For this review, take the finished solid that the model builds, in its own axes (mm). A direction names the side the tool comes from. Coordinates: 2 decimals unless noted, no trailing zeros. Order: outer loops, then holes, each group sorted by start corner. A loop starts at its lowest first (then second) coordinate and runs counter-clockwise, first axis right, second up. Notation, with made-up numbers: (84.25, -4) - (120.25, -4) arc R19 ccw to (120.25, 19) - close; hole circle Ø4 at (12, -7). An arc over 180 degrees is marked (long way). One line per item, written item: value. Start each with the question number.
(1) Consider section D-D on y = -26. Write out the cut boundary in (x, z).
(2) To check wall thickness, follow line 1 along Z through (x, y) = (-56.5, 14.5); line 2 along X through (y, z) = (1, 28); line 3 along X through (y, z) = (2, 11). State the ranges of each line that lie inside material, in increasing order.
(3) Consider section A-A on y = 0. Write out the cut boundary in (x, z).
(4) Consider section C-C on z = 21.5. Write out the cut boundary in (x, y), then the cut area to 3 significant figures.
(5) Consider section B-B on x = -55. Write out the cut boundary in (y, z), then the cut area to 3 significant figures.
(6) Clearance check with flat-ended pins moving along their axes: pin 1 (6 mm diameter, centred on x = 5, y = -17, fed in from -Z); pin 2 (21 mm diameter, centred on x = -18.5, y = 5.5, fed in from +Z); pin 3 (12 mm diameter, centred on y = -4.5, z = 22, fed in from +X). State where each tip first meets the part, or that it passes through.
(7) Mouldability with a two-part tool opening along Y and no side actions: class faces 1 (the flat face through (60, 0, 53.848)), 2 (the cylindrical face through (63.58, 0.98, 28.48)), 3 (the cylindrical face through (63.58, 0.98, 0.63)) as released by +Y, released by -Y, zero draft, split by the parting line, or undercut.
(8) For faces 4 (the flat face through (0, 5, 1.27)), 5 (the flat face through (0, 39.716, 2)), 6 (the cylindrical face through (-63.075, 0.142, 28.479)), list the 3-axis set-ups (+Z, -Z, +X, -X, +Y, -Y) from which the entire face can be reached by the end or side of a thin tool; tool diameter is ignored.
```python
from build123d import *

# Parameters (mm, degrees)
F0_W     = 134.956628
F0_H     = 69.98465
F1_DEPTH = 3.81
F2_T     = -2.54
F3_R     = 3.221336
F3_R_2   = 3.263541
F4_DEPTH = 53.848


with BuildPart() as f1:
    # F0 (on Top) → F1 (new body)
    with BuildSketch(Plane.XY):
        with Locations((1.349568, 4.723483)):
            Rectangle(F0_W, F0_H)
    extrude(amount=F1_DEPTH)

    # F2
    f2_openings = [f1.faces().sort_by_distance(p)[0] for p in [
        (1.349568, 4.723483, 0),
    ]]
    offset(amount=F2_T, openings=f2_openings)

    # F3 (on Top) → F4 (join)
    with BuildSketch(Plane.XY):
        with Locations((-59.856646, 0)):
            Circle(F3_R)
        with Locations((60.466468, 0)):
            Circle(F3_R_2)
    extrude(amount=F4_DEPTH)


solid = f1.part
```
Geometry check:
1. outline: (-66.13, 0) - (-63.59, 0) - (-63.59, 1.27) - (66.29, 1.27) - (66.29, 0) - (68.83, 0) - (68.83, 3.81) - (-66.13, 3.81) - close
2. line 1: z = 1.27 to 3.81
2. line 2: x = -62.92 to -56.79, 57.36 to 63.57
2. line 3: x = -62.38 to -57.33, 57.89 to 63.05
3. outline: (-66.13, 0) - (-63.59, 0) - (-63.59, 1.27) - (-63.08, 1.27) - (-63.08, 0) - (-56.64, 0) - (-56.64, 1.27) - (57.2, 1.27) - (57.2, 0) - (63.73, 0) - (63.73, 1.27) - (66.29, 1.27) - (66.29, 0) - (68.83, 0) - (68.83, 3.81) - (63.73, 3.81) - (63.73, 53.85) - (57.2, 53.85) - (57.2, 3.81) - (-56.64, 3.81) - (-56.64, 53.85) - (-63.08, 53.85) - (-63.08, 3.81) - (-66.13, 3.81) - close
4. outline: circle Ø6.44 at (-59.86, 0); circle Ø6.53 at (60.47, 0)
4. area: 66.1 mm^2
5. outline: (-30.27, 0) - (-27.73, 0) - (-27.73, 1.27) - (37.18, 1.27) - (37.18, 0) - (39.72, 0) - (39.72, 3.81) - (-30.27, 3.81) - close
5. area: 184 mm^2
6. pin 1: stops at z = 1.27
6. pin 2: stops at z = 3.81
6. pin 3: stops at x = 63.73
7. face 1: zero draft
7. face 2: split by the parting line
7. face 3: undercut
8. face 4: -Z
8. face 5: +Z, -Z, +X, -X, +Y
8. face 6: +Z
